Job drawing, mm, ordinate dimensions from the low corner. One solid piece. A direction names the side the tool comes from. Coordinates: 2 decimals unless noted, no trailing zeros. Order: outer loops, then holes, each group sorted by start corner. A loop starts at its lowest first (then second) coordinate and runs counter-clockwise, first axis right, second up. Notation, with made-up numbers: (27, 61) - (45, 61) arc R25 cw to (45, 74) - close; hole circle Ø2 at (54.25, 79). An arc over 180 degrees is marked (long way). Use one line per item in the form item = value.
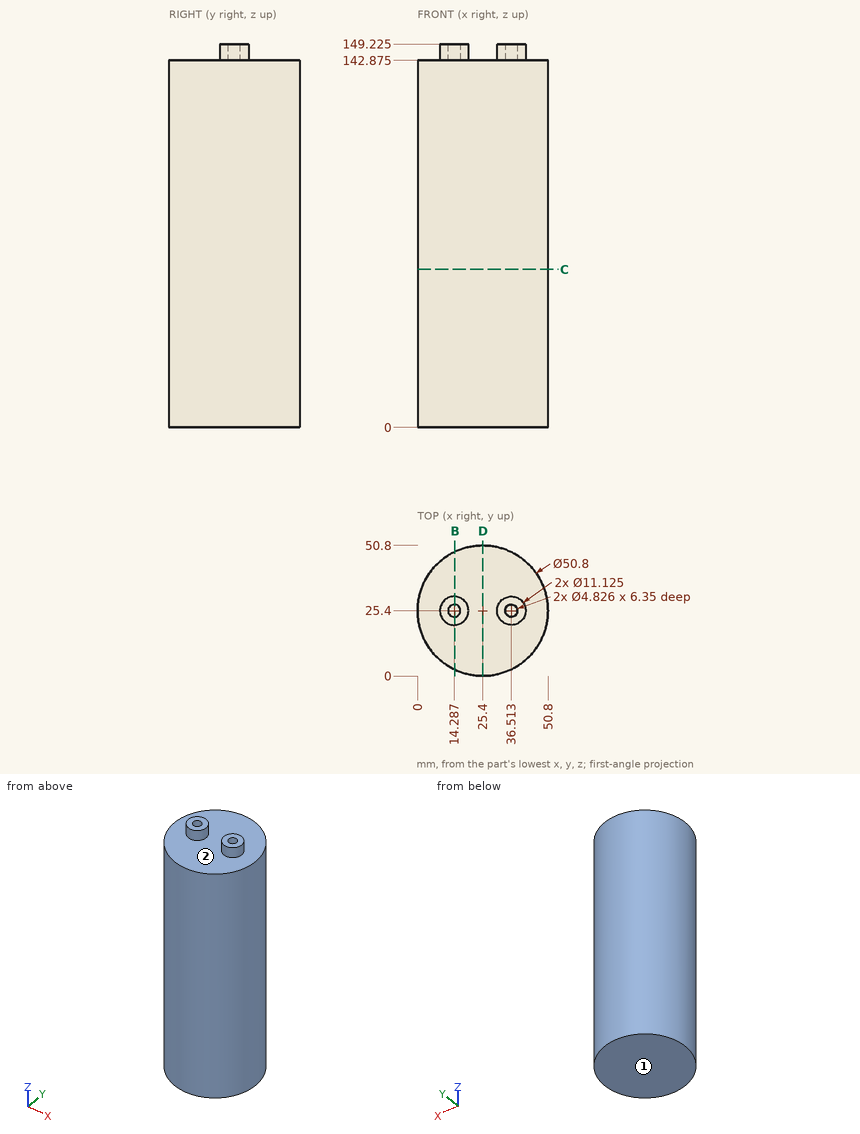
Item 1: Cut at B-B, the plane x = 14.5. Write the cut outline in (y, z) (1 decimal).
Derived:
outline = (2.5, 0) - (48.3, 0) - (48.3, 142.9) - (31, 142.9) - (31, 149.2) - (27.8, 149.2) - (27.8, 142.9) - (23, 142.9) - (23, 149.2) - (19.8, 149.2) - (19.8, 142.9) - (2.5, 142.9) - close
Item 2: Drill centre lines: line 1 (X direction, y = 25, z = 146) (1 decimal); line 2 (Z direction, x = 48, y = 30) (1 decimal); line 3 (X direction, y = 25, z = 37). Where is each one in solid material? Low to high. Write a range as [from, to].
Derived:
line_1 = [8.7, 11.9], [16.7, 19.8], [31, 34.1], [38.9, 42.1]
line_2 = [0, 142.9]
line_3 = [0, 50.8]
Item 3: Drop flat-ended pins along their axis: pin 1 (8 mm diameter, centred on x = 32.5, z = 117, fed in from -Y); pin 2 (1 mm diameter, centred on x = 27.5, y = 15.5, fed in from +Z) (1 decimal); pin 3 (4 mm diameter, centred on y = 34, z = 45.5, fed in from +X). Give the stop position or say it passes through.
Derived:
pin_1 = 0.19
pin_2 = 142.9
pin_3 = 49.93
Item 4: Cut at D-D, the plane x = 25.4. Write the cut outline in (y, z) (1 decimal).
Derived:
outline = (0, 0) - (50.8, 0) - (50.8, 142.9) - (0, 142.9) - close
Item 5: 3-axis set-ups, long thin cutter, end or side, ignore diameter. For the marked faces 1 and 2: which of +Z, -Z, +X, -X, +Y, -Y reach the whole face in a straight line?
Derived:
face_1 = -Z, +X, -X, +Y, -Y
face_2 = +Z
Item 6: Cut at C-C, the plane z = 61.5. Write the cut outline in (x, y), plus the area to 3 significant figures.
Derived:
outline = circle Ø50.8 at (25.4, 25.4)
area = 2,030 mm²
